```python
from build123d import *

# Parameters (mm, degrees)
CROQUIS1_W              = 44
CROQUIS1_H              = 20
SALIENTE_EXTRUIR1_DEPTH = 2
CROQUIS2_R              = 3
CROQUIS2_R_2            = 1.5
CORTAR_EXTRUIR1_DEPTH   = 2
CROQUIS3_W              = 2
CROQUIS3_H              = 20
SALIENTE_EXTRUIR2_DEPTH = 25
REDONDEO1_R             = 10
REDONDEO2_R             = 2
CORTAR_EXTRUIR2_REACH   = 54.583
CROQUIS4_R              = 4


with BuildPart() as part:
    # Croquis1 → Saliente-Extruir1 (new body)
    with BuildSketch(Plane.XY):
        Rectangle(CROQUIS1_W, CROQUIS1_H)
    extrude(amount=SALIENTE_EXTRUIR1_DEPTH)

    # Croquis2 → Cortar-Extruir1 (cut)
    with BuildSketch(Plane.XY.offset(2)):
        Circle(CROQUIS2_R)
        with Locations((-4.949747468, 4.949747468)):
            Circle(CROQUIS2_R_2)
        with Locations(Location((4.949747468, 4.949747468, 0), (0, 0, 180))):
            Circle(CROQUIS2_R_2)
        with Locations((4.949747468, -4.949747468)):
            Circle(CROQUIS2_R_2)
        with Locations(Location((-4.949747468, -4.949747468, 0), (0, 0, 180))):
            Circle(CROQUIS2_R_2)
    extrude(amount=-CORTAR_EXTRUIR1_DEPTH, mode=Mode.SUBTRACT)

    # Croquis3 → Saliente-Extruir2 (add)
    with BuildSketch(Plane.XY.offset(2)):
        with Locations((-21, 0)):
            Rectangle(CROQUIS3_W, CROQUIS3_H)
        with Locations((21, 0)):
            Rectangle(CROQUIS3_W, CROQUIS3_H)
    extrude(amount=SALIENTE_EXTRUIR2_DEPTH)

    # Redondeo1
    redondeo1_edges = [part.edges().sort_by_distance(p)[0] for p in [
        (21, 10, 27),
        (21, -10, 27),
    ]]
    fillet(redondeo1_edges, radius=REDONDEO1_R - 0.0001)  # a hair under: the kernel refuses the full size

    # Redondeo2
    redondeo2_edges = [part.edges().sort_by_distance(p)[0] for p in [
        (-21, -10, 27),
        (-21, 10, 27),
    ]]
    fillet(redondeo2_edges, radius=REDONDEO2_R)

    # Cortar-Extruir2: up to this face of the body (flat: up to its plane)
    cortar_extruir2_end = Plane(part.part.faces().sort_by_distance((-22, 0, 13.458367573))[0])
    # Croquis4 → Cortar-Extruir2 (cut, up to the picked face)
    with BuildSketch(Plane(origin=(22, 0, 0), x_dir=(0, 0, -1), z_dir=(1, 0, 0)), mode=Mode.PRIVATE) as cortar_extruir2_sk1:
        with Locations((-17, 0)):
            Circle(CROQUIS4_R)
    cortar_extruir2_tool1 = split(extrude(cortar_extruir2_sk1.sketch, amount=-CORTAR_EXTRUIR2_REACH, mode=Mode.PRIVATE), bisect_by=cortar_extruir2_end, keep=Keep.BOTH, mode=Mode.PRIVATE)
    add(cortar_extruir2_tool1.solids().sort_by(Axis((22, 0, 17), (-1, 0, 0)))[0], mode=Mode.SUBTRACT)


solid = part.part
```
Here's how the part is built. I have some questions about the finished solid (model axes, mm). A direction names the side the tool comes from. Round coordinates to 2 decimals unless told otherwise and drop trailing zeros. Order: outer loops, then holes, each group sorted by start corner. A loop starts at its lowest first (then second) coordinate and runs counter-clockwise, first axis right, second up. Notation, with made-up numbers: (58, 15) -> (86, 15) arc R15 cw to (86, 21) -> close; hole circle Ø2 at (-38, 19.5). An arc over 180 degrees is marked (long way). Use a Markdown table: item, result. Add a question column.
(1) Suppose I cut it at D-D, the plane y = -7. Please give me the cut outline in (x, z), and give its area (3 significant figures).
(2) I need wall thicknesses on line 1 along X through (y, z) = (-1.5, 10.25); line 2 along Z through (x, y) = (6.5, -0.5). Which ranges of each line are inside material? Lowest first, please.
(3) Suppose I cut it at A-A, the plane z = 9.5. Please give me the cut outline in (x, y), and give its area (3 significant figures).
(4) If we mould it in two halves opening along Z, with no side actions, what happens to faces 6 (the face through (-21, -2.4, 20.2)), 7 (the face through (-21, 0, 27)), 8 (the face through (21, -2.4, 20.2)), 9 (the face through (-22, -2, 13))? For each: released by +Z, released by -Z, zero draft, split by the parting line, or undercut.
(5) Suppose I cut it at C-C, the plane y = -2.5. Please give me the cut outline in (x, z).
(6) For pin 1 Ø4 at (x, y) = (-5.5, 5) entering from +Z, with a flat end and sliding along its axis, tell me the tip position at first contact or that it passes through.
(7) Suppose I cut it at B-B, the plane x = 0. Please give me the cut outline in (y, z).
(8) For faces 1 (the face through (20, 0, 12)), 2 (the face through (5.756, -3.685, 1.014)), 3 (the face through (-2, 10, 1)), 4 (the face through (21.01, 6.99, 24.15)), 5 (the face through (21.01, -7.15, 23.99)), which set-ups out of +Z, -Z, +X, -X, +Y, -Y let a thin tool reach every point of the face, with its end or its side?
Verdict:
| question | item | result |
|---|---|---|
| 1 | outline | (-22, 0) -> (22, 0) -> (22, 24.14) -> (20, 24.14) -> (20, 2) -> (-20, 2) -> (-20, 27) -> (-22, 27) -> close |
| 1 | area | 182 mm2 |
| 2 | line 1 | -22 to -20, 20 to 22 |
| 2 | line 2 | 0 to 2 |
| 3 | outline | (-22, -10) -> (-20, -10) -> (-20, 10) -> (-22, 10) -> close; (20, -10) -> (22, -10) -> (22, 10) -> (20, 10) -> close |
| 3 | area | 80.0 mm2 |
| 4 | face 6 | undercut |
| 4 | face 7 | released by +Z |
| 4 | face 8 | undercut |
| 4 | face 9 | zero draft |
| 5 | outline | (-22, 0) -> (-1.66, 0) -> (-1.66, 2) -> (-20, 2) -> (-20, 13.88) -> (-22, 13.88) -> close; (-22, 20.12) -> (-20, 20.12) -> (-20, 27) -> (-22, 27) -> close; (1.66, 0) -> (22, 0) -> (22, 13.88) -> (20, 13.88) -> (20, 2) -> (1.66, 2) -> close; (20, 20.12) -> (22, 20.12) -> (22, 26.68) -> (20, 26.68) -> close |
| 6 | pin 1 | z = 2 |
| 7 | outline | (-10, 0) -> (-3, 0) -> (-3, 2) -> (-10, 2) -> close; (3, 0) -> (10, 0) -> (10, 2) -> (3, 2) -> close |
| 8 | face 1 | +Z, +Y, -Y |
| 8 | face 2 | +Z, -Z |
| 8 | face 3 | +Z, -Z, +X, -X, +Y |
| 8 | face 4 | +Z, +X, +Y |
| 8 | face 5 | +Z, +X, -Y |
